from build123d import *

# Parameters (mm, degrees)
SKETCH1_R           = 1.397
SKETCH1_W           = 3.175
SKETCH1_H           = 4.953
SKETCH1_W_2         = 11.43
SKETCH1_H_2         = 3.048
SKETCH1_W_3         = 43.434
BOSS_EXTRUDE1_DEPTH = 3.048
FILLET1_R           = 2.54
SKETCH2_R           = 2
BOSS_EXTRUDE2_DEPTH = 3.048


with BuildPart() as part:
    # Sketch1 → Boss-Extrude1 (new body)
    with BuildSketch(Plane.XY):
        Polygon((-3.7846, 71.611586257), (-3.7846, -5.588), (21.3106, -5.588), (21.3106, -4.3434), (21.3106, 8.255), (16.256, 8.255), (16.256, 15.1384), (38.7858, 15.1384), (38.7858, -4.3434), (38.7858, -5.588), (63.5254, -5.588), (63.5254, 71.611586257), align=None)
        with Locations((5.3594, 3.556)):
            Circle(SKETCH1_R, mode=Mode.SUBTRACT)
        with Locations((9.8171, 10.8077)):
            Rectangle(SKETCH1_W, SKETCH1_H, mode=Mode.SUBTRACT)
        with Locations((13.8684, -1.524)):
            Rectangle(SKETCH1_W_2, SKETCH1_H_2, mode=Mode.SUBTRACT)
        with Locations((45.8724, -1.524)):
            Rectangle(SKETCH1_W_2, SKETCH1_H_2, mode=Mode.SUBTRACT)
        with Locations((54.3814, 3.556)):
            Circle(SKETCH1_R, mode=Mode.SUBTRACT)
        with BuildLine():
            Line((-1.2446, 63.754), (1.8034, 63.754))
            Line((1.8034, 63.754), (1.8034, 58.42))
            Line((1.8034, 58.42), (5.3594, 58.42))
            ThreePointArc((5.3594, 58.42), (7.60446403, 59.34993597), (8.5344, 61.595))
            Line((8.5344, 61.595), (51.2064, 61.595))
            ThreePointArc((51.2064, 61.595), (52.13633597, 59.34993597), (54.3814, 58.42))
            Line((54.3814, 58.42), (57.9374, 58.42))
            Line((57.9374, 58.42), (57.9374, 63.754))
            Line((57.9374, 63.754), (60.9854, 63.754))
            Line((60.9854, 63.754), (60.9854, 3.2766))
            Line((60.9854, 3.2766), (57.9374, 3.2766))
            Line((57.9374, 3.2766), (57.9374, 6.731))
            Line((57.9374, 6.731), (51.2064, 6.731))
            Line((51.2064, 6.731), (51.2064, 21.7424))
            Line((51.2064, 21.7424), (1.8034, 21.7424))
            Line((1.8034, 21.7424), (1.8034, 3.2766))
            Line((1.8034, 3.2766), (-1.2446, 3.2766))
            Line((-1.2446, 3.2766), (-1.2446, 63.754))
        make_face(mode=Mode.SUBTRACT)
        with Locations((5.3594, 61.595)):
            Circle(SKETCH1_R, mode=Mode.SUBTRACT)
        with Locations((29.8704, 66.294)):
            Rectangle(SKETCH1_W_3, SKETCH1_H_2, mode=Mode.SUBTRACT)
        with Locations((54.3814, 61.595)):
            Circle(SKETCH1_R, mode=Mode.SUBTRACT)
    extrude(amount=BOSS_EXTRUDE1_DEPTH)

    # Fillet1
    fillet1_edges = [part.edges().sort_by_distance(p)[0] for p in [
        (-3.7846, -5.588, 1.524),
        (-3.7846, 71.611586257, 1.524),
        (63.5254, 71.611586257, 1.524),
        (63.5254, -5.588, 1.524),
    ]]
    fillet(fillet1_edges, radius=FILLET1_R)

    # Sketch2 → Boss-Extrude2 (add)
    with BuildSketch(Plane.XY.offset(3.048)):
        with BuildLine():
            ThreePointArc((-3.055036152, 70.853136408), (-2.226043482, 71.414313021), (-1.2446, 71.611586257))
            Line((-1.2446, 71.611586257), (-5.010493887, 74.127944533))
            ThreePointArc((-5.010493887, 74.127944533), (-11.175901405, 72.901649241), (-9.949606113, 66.736241724))
            Line((-9.949606113, 66.736241724), (-3.7846, 62.616804315))
            Line((-3.7846, 62.616804315), (-3.7846, 67.961936393))
            ThreePointArc((-3.7846, 67.961936393), (-3.170149461, 69.344535157), (-3.055036152, 70.853136408))
        make_face()
        with Locations((-7.48005, 70.432093129)):
            Circle(SKETCH2_R, mode=Mode.SUBTRACT)
        with BuildLine():
            ThreePointArc((-1.2446, -5.588), (-2.226043482, -5.390726764), (-3.055036152, -4.829550151))
            ThreePointArc((-3.055036152, -4.829550151), (-3.170149461, -3.3209489), (-3.7846, -1.938350136))
            Line((-3.7846, -1.938350136), (-3.7846, 3.406781942))
            Line((-3.7846, 3.406781942), (-9.949606113, -0.712655467))
            ThreePointArc((-9.949606113, -0.712655467), (-11.175901405, -6.878062984), (-5.010493887, -8.104358276))
            Line((-5.010493887, -8.104358276), (-1.2446, -5.588))
        make_face()
        with Locations((-7.48005, -4.408506871)):
            Circle(SKETCH2_R, mode=Mode.SUBTRACT)
        with BuildLine():
            ThreePointArc((64.751293887, -8.104358276), (70.916701405, -6.878062984), (69.690406113, -0.712655467))
            Line((69.690406113, -0.712655467), (63.5254, 3.406781942))
            Line((63.5254, 3.406781942), (63.5254, -1.938350136))
            ThreePointArc((63.5254, -1.938350136), (62.910949461, -3.3209489), (62.795836152, -4.829550151))
            ThreePointArc((62.795836152, -4.829550151), (61.966843482, -5.390726764), (60.9854, -5.588))
            Line((60.9854, -5.588), (64.751293887, -8.104358276))
        make_face()
        with Locations((67.22085, -4.408506871)):
            Circle(SKETCH2_R, mode=Mode.SUBTRACT)
        with BuildLine():
            ThreePointArc((60.9854, 71.611586257), (61.966843482, 71.414313021), (62.795836152, 70.853136408))
            ThreePointArc((62.795836152, 70.853136408), (62.910949461, 69.344535157), (63.5254, 67.961936393))
            Line((63.5254, 67.961936393), (63.5254, 62.616804315))
            Line((63.5254, 62.616804315), (69.690406113, 66.736241724))
            ThreePointArc((69.690406113, 66.736241724), (70.916701405, 72.901649241), (64.751293887, 74.127944533))
            Line((64.751293887, 74.127944533), (60.9854, 71.611586257))
        make_face()
        with Locations((67.22085, 70.432093129)):
            Circle(SKETCH2_R, mode=Mode.SUBTRACT)
    extrude(amount=-BOSS_EXTRUDE2_DEPTH)


solid = part.part
The listing builds one solid part. Answer for the finished solid, in the listing's coordinates (mm). A direction names the side the tool comes from. Give positions to 0.01 mm unless a question says otherwise; leave off trailing zeros. Write each loop counter-clockwise with the first axis right and the second up, starting at its lowest first coordinate (ties: lowest second). Pieces come first, ordered by that corner, then holes.
Item 1: Flat-ended cylindrical pins translate along their axes: P1, Ø0.9, axis at y = 10.5, z = 1.5, coming from the +X side; P2, Ø1.5, axis at x = 59, z = 1, coming from the +Y side; P3, Ø1.5, axis at x = 56, z = 1.5, coming from the -Y side; P4, Ø2.5, axis at x = -7.48, y = -4.41, coming from the +Z side. Find the tip coordinate at first contact, or state that the pin passes through.
Item 2: Section B-B, the plane y = 19 is taken. Write down the section's boundary in (x, z).
Item 3: Determine the mould class of faces 1 (the flat face through (-6.82, 1.38, 1.55)), 2 (the flat face through (27, 21, 0)), 3 (the flat face through (14, 0, 2)), 4 (the flat face through (1.803, 13, 2)) for opening direction X: released by +X, released by -X, zero draft, split by the parting line, or undercut.
Item 4: Section D-D, the plane y = 42 is taken. Write down the section's boundary in (x, z).
Item 5: Find the intervals of material crossed by line 1 along Y through (x, z) = (36, 2.1) (3 decimals); line 2 along Y through (x, z) = (21, 1) (3 decimals); line 3 along Y through (x, z) = (16.5, 2) (3 decimals), in increasing order.
Item 6: Which of the six approach directions +Z, -Z, +X, -X, +Y, -Y give full straight-line access (tool end or side, diameter ignored) to faces 5 (the flat face through (-3.1, 72.85, 1.55)), 6 (the flat face through (-6.9, 64.7, 1.5)), 7 (the flat face through (4, 58.42, 2)), 8 (the flat face through (62.8, -6.8, 1.5))?
Item 7: Section C-C, the plane x = 31.5 is taken. Write down the section's boundary in (y, z) (3 decimals), plus the area to 3 significant figures.
Item 8: Section A-A, the plane x = 0 is taken. Write down the section's boundary in (y, z), plus the area to 3 significant figures.
Completed:
1. P1: stops at x = 63.53
1. P2: stops at y = 71.61
1. P3: stops at y = -5.59
1. P4: passes through
2. outline: (-3.78, 0) - (-1.24, 0) - (-1.24, 3.05) - (-3.78, 3.05) - close; (1.8, 0) - (51.21, 0) - (51.21, 3.05) - (1.8, 3.05) - close; (60.99, 0) - (63.53, 0) - (63.53, 3.05) - (60.99, 3.05) - close
3. face 1: released by -X
3. face 2: zero draft
3. face 3: undercut
3. face 4: undercut
4. outline: (-3.78, 0) - (-1.24, 0) - (-1.24, 3.05) - (-3.78, 3.05) - close; (60.99, 0) - (63.53, 0) - (63.53, 3.05) - (60.99, 3.05) - close
5. line 1: y = 15.138 to 21.742, 61.595 to 64.77, 67.818 to 71.612
5. line 2: y = -5.588 to 8.255, 15.138 to 21.742, 61.595 to 64.77, 67.818 to 71.612
5. line 3: y = -5.588 to -3.048, 0 to 8.255, 15.138 to 21.742, 61.595 to 64.77, 67.818 to 71.612
6. face 5: +Z, -Z, +Y
6. face 6: +Z, -Z, -X
6. face 7: +Z, -Z
6. face 8: +Z, -Z, -Y
7. outline: (15.138, 0) - (21.742, 0) - (21.742, 3.048) - (15.138, 3.048) - close; (61.595, 0) - (64.77, 0) - (64.77, 3.048) - (61.595, 3.048) - close; (67.818, 0) - (71.612, 0) - (71.612, 3.048) - (67.818, 3.048) - close
7. area: 41.4 mm2
8. outline: (-5.59, 0) - (3.28, 0) - (3.28, 3.05) - (-5.59, 3.05) - close; (63.75, 0) - (71.61, 0) - (71.61, 3.05) - (63.75, 3.05) - close
8. area: 51.0 mm2
